For this review, take the finished solid that the model builds, in its own axes (mm). A direction names the side the tool comes from. Round coordinates to 2 decimals unless told otherwise and drop trailing zeros. Write each loop counter-clockwise with the first axis right and the second up, starting at its lowest first coordinate (ties: lowest second). Pieces come first, ordered by that corner, then holes. Notation, with made-up numbers: (-34, -27.5) -> (-18, -27.5) arc R27 ccw to (-18, -3.5) -> close; hole circle Ø4 at (76.25, 71.5). An arc over 180 degrees is marked (long way). Write item = value, one per line. Start each with the question number.
Autodesk Inventor part; units mm, degrees
ref_plane "YZ Plane" through (0, 0, 0) normal (1, 0, 0) x (0, 1, 0)
ref_plane "XZ Plane" through (0, 0, 0) normal (0, 1, 0) x (-1, 0, 0)
ref_plane "XY Plane" through (0, 0, 0) normal (0, 0, 1) x (1, 0, 0)
sketch "Sketch1" plane through (0, 0, 0) normal (0, 0, 1) x (1, 0, 0)
  line L0 (-12.5, 12.5) -> (12.5, 12.5)
  line L1 (12.5, 12.5) -> (12.5, -12.5)
  line L2 (12.5, -12.5) -> (-12.5, -12.5)
  line L3 (-12.5, -12.5) -> (-12.5, 12.5)
  line L4 (-12.5, 12.5) -> (12.5, -12.5) construction
  line L5 (-12.5, -12.5) -> (12.5, 12.5) construction
  arc A0 (-1.7861, 2.625) -> (1.7861, 2.625) centre (0, 0) ccw
  line L6 (-1.7861, 2.625) -> (1.7861, 2.625)
  circle A1 centre (-6.5, 6.5) radius 2.5
  circle A2 centre (6.5, 6.5) radius 2.5
  circle A3 centre (6.5, -6.5) radius 2.5
  circle A4 centre (-6.5, -6.5) radius 2.5
  line L7 (1.9339, 3.125) -> (-1.9339, 3.125)
  arc A5 (-1.9339, 3.125) -> (1.9339, 3.125) centre (0, 0) ccw
  point P0 (0, 0)
  dimension "d0" = 6.35
  dimension "d1" = 25
  dimension "d2" = 5.8
  dimension "d3" = 5
  dimension "d6" = 13
  dimension "d7" = 0.5
extrude "Extrusion1" add sketch "Sketch1" along normal blind 3 contours L0 L1 L2 L3
sketch "Sketch2" plane through (0, 0, 3) normal (0, 0, 1) x (1, 0, 0)
  line L0 (12.5, 12.5) -> (-12.5, 12.5)
  line L1 (-12.5, 12.5) -> (-12.5, -12.5)
  line L2 (-12.5, -12.5) -> (12.5, -12.5)
  line L3 (12.5, -12.5) -> (12.5, 12.5)
  circle A0 centre (-6.5, 6.5) radius 2.5
  circle A1 centre (6.5, 6.5) radius 2.5
  circle A2 centre (6.5, -6.5) radius 2.5
  circle A3 centre (-6.5, -6.5) radius 2.5
  arc A4 (-1.9339, 3.125) -> (1.9339, 3.125) centre (0, 0) ccw
  line L4 (-1.9339, 3.125) -> (1.9339, 3.125)
  arc A5 (-2.8723, 7.2281) -> (-7.2281, 2.8723) centre (-6.5, 6.5) ccw
  arc A6 (-7.2281, -2.8723) -> (-2.8723, -7.2281) centre (-6.5, -6.5) ccw
  arc A7 (2.8723, -7.2281) -> (7.2281, -2.8723) centre (6.5, -6.5) ccw
  arc A8 (7.2281, 2.8723) -> (2.8723, 7.2281) centre (6.5, 6.5) ccw
  arc A9 (-7.2281, -2.8723) -> (-7.2281, 2.8723) centre (-7.8046, 0) ccw
  arc A10 (-2.8723, 7.2281) -> (2.8723, 7.2281) centre (0, 7.8046) ccw
  arc A11 (7.2281, 2.8723) -> (7.2281, -2.8723) centre (7.8046, 0) ccw
  arc A12 (2.8723, -7.2281) -> (-2.8723, -7.2281) centre (0, -7.8046) ccw
  point P0 (0, 0)
  dimension "d12" = 1.2
  dimension "d13" = 1.2
extrude "Extrusion2" cut sketch "Sketch2" against normal through all contours L3 L2 L1 L0
sketch "Sketch3" plane through (0, 0, 3) normal (0, 0, 1) x (1, 0, 0)
  arc A0 (-2.8723, 7.2281) -> (-7.2281, 2.8723) centre (-6.5, 6.5) ccw
  arc A1 (-7.2281, -2.8723) -> (-7.2281, 2.8723) centre (-7.8046, 0) ccw
  arc A2 (-7.2281, -2.8723) -> (-2.8723, -7.2281) centre (-6.5, -6.5) ccw
  arc A3 (2.8723, -7.2281) -> (-2.8723, -7.2281) centre (0, -7.8046) ccw
  arc A4 (2.8723, -7.2281) -> (7.2281, -2.8723) centre (6.5, -6.5) ccw
  arc A5 (7.2281, 2.8723) -> (7.2281, -2.8723) centre (7.8046, 0) ccw
  arc A6 (7.2281, 2.8723) -> (2.8723, 7.2281) centre (6.5, 6.5) ccw
  arc A7 (-2.8723, 7.2281) -> (2.8723, 7.2281) centre (0, 7.8046) ccw
  circle A8 centre (-6.5, 6.5) radius 2.5
  circle A9 centre (6.5, 6.5) radius 2.5
  circle A10 centre (6.5, -6.5) radius 2.5
  circle A11 centre (-6.5, -6.5) radius 2.5
  arc A12 (-1.9339, 3.125) -> (1.9339, 3.125) centre (0, 0) ccw
  line L0 (-1.9339, 3.125) -> (1.9339, 3.125)
  circle A13 centre (0, 0) radius 4.875
  arc A14 (-7.2281, -2.8723) -> (-7.2281, 2.8723) centre (-7.8046, 0) ccw
  point P0 (0, 0)
extrude "Extrusion3" add sketch "Sketch3" along normal blind 12 contours A13
chamfer "Chamfer1" distance 0.5 angle 45 2 edges at (0, 3.125, 15) (0, -3.675, 15)
properties part number "teenee_part"
1. Clearance check with flat-ended pins moving along their axes: pin 1 Ø6 at (x, y) = (0, 0) entering from +Z; pin 2 Ø1.5 at (y, z) = (2.5, 13) entering from +X; pin 3 Ø6 at (x, y) = (2, 4.5) entering from +Z; pin 4 Ø8 at (x, y) = (6.5, 6.5) entering from +Z. State where each tip first meets the part, or that it passes through.
2. Wall thickness on L1, parallel to Y at x = 0, z = 11.75 (3 decimals); L2, parallel to Y at x = 6.5, z = 2; L3, parallel to X at y = -7.5, z = 1: over which ranges is each line inside the solid? List them lowest first. Write a range as from..to.
3. Machinability: for faces 1 (the flat face through (4, 5, 3)), 2 (the flat face through (-5, 4, 3)), 3 (the flat face through (-4, -5, 3)), 4 (the cylindrical face through (-0.635, -4.834, 8.916)), which of the approach directions +Z, -Z, +X, -X, +Y, -Y give a long, thin tool a straight path to every point of the face, cutting with its end or side? Answer none if there is none.
4. Consider section A-A, the plane x = -6.5. Give the boundary of the cut face in (y, z), then the cut area to 3 significant figures.
5. Consider section C-C, the plane z = 10. Give the boundary of the cut face in (x, y) (3 decimals), then the cut area to 3 significant figures.
6. Draft analysis for pull direction Y (two halves, no side actions). For faces 5 (the cylindrical face through (-4.115, 5.749, 1.479)), 6 (the flat face through (1, 4, 15)), 7 (the cylindrical face through (0.056, -4.876, 1.521)), state which applies: +Y half, -Y half, draft (parallel to the pull), parting line (faces both ways), or undercut.
Outcome:
q1.pin_1 = through
q1.pin_2 = 4.55
q1.pin_3 = 15
q1.pin_4 = 3
q2.L1 = -4.875..-3.675, 3.125..4.875
q2.L2 = -10.2..-9, -4..-2.62, 2.62..4, 9..10.2
q2.L3 = -10.06..-8.79, -4.21..-2.94, 2.94..4.21, 8.79..10.06
q3.face_1 = +Z, +X, +Y
q3.face_2 = +Z, -X, +Y
q3.face_3 = +Z, -X, -Y
q3.face_4 = +Z
q4.outline = (-10.2, 0) -> (-9, 0) -> (-9, 3) -> (-10.2, 3) -> close; (-4, 0) -> (-2.62, 0) -> (-2.62, 3) -> (-4, 3) -> close; (2.62, 0) -> (4, 0) -> (4, 3) -> (2.62, 3) -> close; (9, 0) -> (10.2, 0) -> (10.2, 3) -> (9, 3) -> close
q4.area = 15.5 mm2
q5.outline = circle Ø9.75 at (0, 0); hole (-1.934, 3.125) arc R3.675 ccw (long way) to (1.934, 3.125) -> close
q5.area = 33.7 mm2
q6.face_5 = undercut
q6.face_6 = draft
q6.face_7 = -Y half
